Print and shaded views of the part. All mm, measured from the part's lowest x, y and z. Coordinates: 2 decimals unless noted, no trailing zeros. Order: outer loops, then holes, each group sorted by start corner. A loop starts at its lowest first (then second) coordinate and runs counter-clockwise, first axis right, second up. Notation, with made-up numbers: (-16.5, 40) - (3.5, 40) arc R15 cw to (3.5, 55) - close; hole circle Ø2 at (53, -18.5). An arc over 180 degrees is marked (long way). Write each question's results on one line, items separated by ' | '.
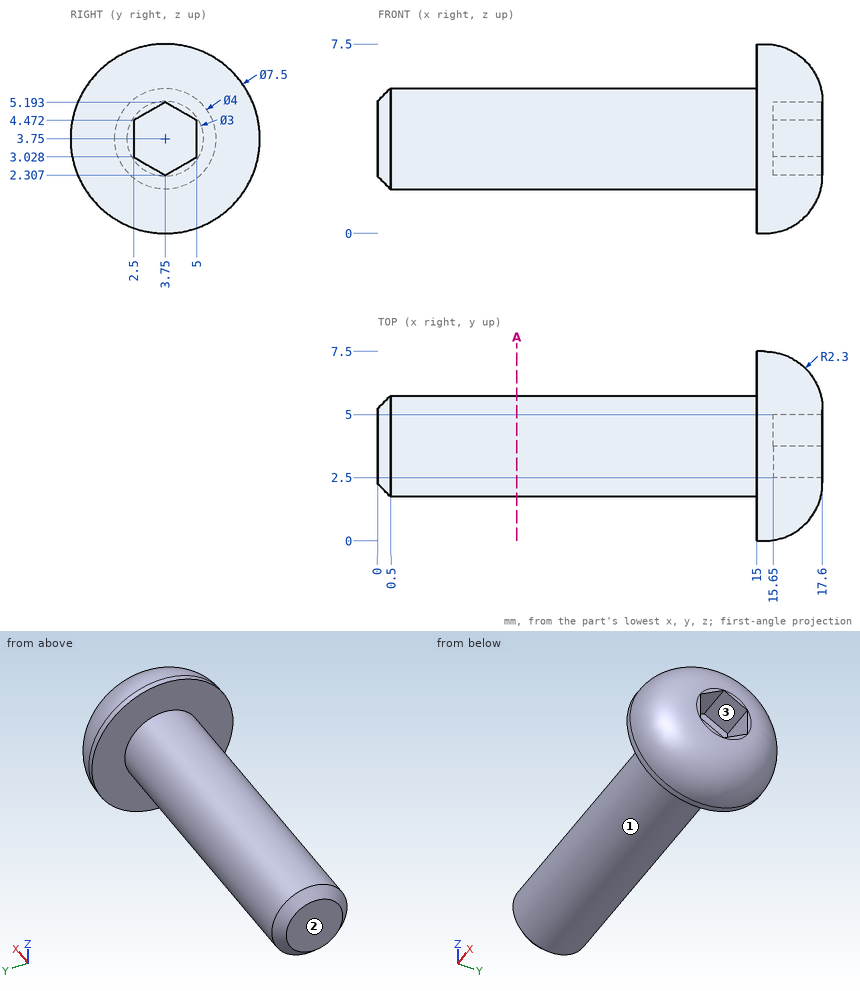
1. Probe line 1 (X direction, y = 3, z = 4); line 2 (Z direction, x = 5.5, y = 2.75); line 3 (Y direction, x = 2, z = 5). List the from-to ranges inside material, lowest first.
Solved:
line 1: x = 0 to 15.65 | line 2: z = 2.02 to 5.48 | line 3: y = 2.19 to 5.31
2. Two-plate mould, pull along Y, no slides. Class the marked faces 1, 2 and 3: +Y half, -Y half, draft (parallel to the pull), parting line (faces both ways), or undercut.
Solved:
face 1: parting line | face 2: draft | face 3: undercut
3. Band-saw the part on A-A on x = 5.5. Give the cut face in (y, z), then the cut area to 3 significant figures.
Solved:
outline: circle Ø4 at (3.75, 3.75) | area: 12.6 mm2
4. Drop flat-ended pins along their axis: pin 1 Ø1.2 at (y, z) = (3.5, 3.5) entering from +X; pin 2 Ø4 at (x, y) = (11, 4) entering from -Z. Give the stop position or say it passes through.
Solved:
pin 1: stops at x = 15.65 | pin 2: stops at z = 1.75
